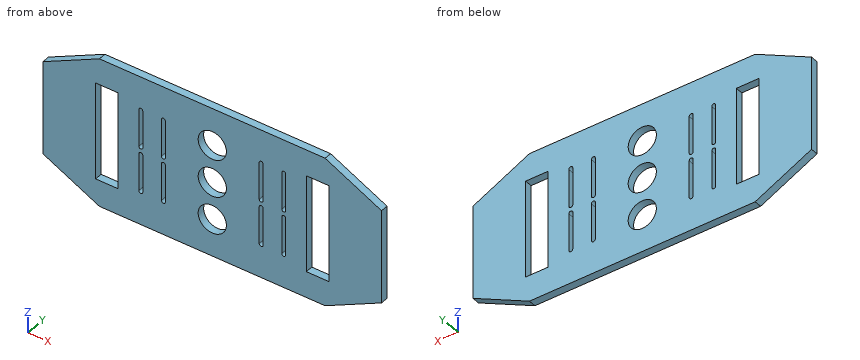
from build123d import *

# Parameters (mm, degrees)
ESQUISSE1_W             = 180
ESQUISSE1_H             = 80
BOSS_EXTRU_1_DEPTH      = 4
ENL_V_MAT_EXTRU_2_DEPTH = 4
ENL_V_MAT_EXTRU_3_DEPTH = 4
ENL_V_MAT_EXTRU_4_REACH = 6
ESQUISSE8_W             = 12
ESQUISSE8_H             = 52
ENL_V_MAT_EXTRU_5_REACH = 6
ESQUISSE9_R             = 7.5


with BuildPart() as part:
    # Esquisse1 → Boss.-Extru.1 (new body)
    with BuildSketch(Plane(origin=(0, 0, 0), x_dir=(1, 0, 0), z_dir=(0, 1, 0))):
        with Locations((90, 40)):
            Rectangle(ESQUISSE1_W, ESQUISSE1_H)
    extrude(amount=BOSS_EXTRU_1_DEPTH)

    # Esquisse2 → Enlèv. mat.-Extru.2 (cut)
    with BuildSketch(Plane(origin=(0, 4, 0), x_dir=(1, 0, 0), z_dir=(0, 1, 0))):
        Polygon((0, 65), (30, 80), (0, 80), align=None)
        Polygon((150, 80), (180, 65), (180, 80), align=None)
        Polygon((150, 0), (180, 15), (180, 0), align=None)
        Polygon((0, 15), (30, 0), (0, 0), align=None)
    extrude(amount=-ENL_V_MAT_EXTRU_2_DEPTH, mode=Mode.SUBTRACT)

    # Esquisse7 → Enlèv. mat.-Extru.3 (cut)
    with BuildSketch(Plane(origin=(0, 4, 0), x_dir=(1, 0, 0), z_dir=(0, 1, 0))):
        with BuildLine():
            Line((62.95, 18), (62.95, 38))
            ThreePointArc((62.95, 38), (64, 39.05), (65.05, 38))
            Line((65.05, 38), (65.05, 18))
            ThreePointArc((65.05, 18), (64, 16.95), (62.95, 18))
        make_face()
        with BuildLine():
            Line((50.95, 18), (50.95, 38))
            ThreePointArc((50.95, 38), (52, 39.05), (53.05, 38))
            Line((53.05, 38), (53.05, 18))
            ThreePointArc((53.05, 18), (52, 16.95), (50.95, 18))
        make_face()
        with BuildLine():
            Line((50.95, 42), (50.95, 62))
            ThreePointArc((50.95, 62), (52, 63.05), (53.05, 62))
            Line((53.05, 62), (53.05, 42))
            ThreePointArc((53.05, 42), (52, 40.95), (50.95, 42))
        make_face()
        with BuildLine():
            Line((62.95, 42), (62.95, 62))
            ThreePointArc((62.95, 62), (64, 63.05), (65.05, 62))
            Line((65.05, 62), (65.05, 42))
            ThreePointArc((65.05, 42), (64, 40.95), (62.95, 42))
        make_face()
        with BuildLine():
            Line((117.05, 42), (117.05, 62))
            ThreePointArc((117.05, 62), (116, 63.05), (114.95, 62))
            Line((114.95, 62), (114.95, 42))
            ThreePointArc((114.95, 42), (116, 40.95), (117.05, 42))
        make_face()
        with BuildLine():
            Line((129.05, 42), (129.05, 62))
            ThreePointArc((129.05, 62), (128, 63.05), (126.95, 62))
            Line((126.95, 62), (126.95, 42))
            ThreePointArc((126.95, 42), (128, 40.95), (129.05, 42))
        make_face()
        with BuildLine():
            Line((129.05, 18), (129.05, 38))
            ThreePointArc((129.05, 38), (128, 39.05), (126.95, 38))
            Line((126.95, 38), (126.95, 18))
            ThreePointArc((126.95, 18), (128, 16.95), (129.05, 18))
        make_face()
        with BuildLine():
            Line((117.05, 18), (117.05, 38))
            ThreePointArc((117.05, 38), (116, 39.05), (114.95, 38))
            Line((114.95, 38), (114.95, 18))
            ThreePointArc((114.95, 18), (116, 16.95), (117.05, 18))
        make_face()
    extrude(amount=-ENL_V_MAT_EXTRU_3_DEPTH, mode=Mode.SUBTRACT)

    # Esquisse8 → Enlèv. mat.-Extru.4 (cut, up to next)
    with BuildSketch(Plane(origin=(0, 4, 0), x_dir=(1, 0, 0), z_dir=(0, 1, 0)), mode=Mode.PRIVATE) as enl_v_mat_extru_4_sk1:
        with Locations((146, 40)):
            Rectangle(ESQUISSE8_W, ESQUISSE8_H)
    enl_v_mat_extru_4_tool1 = extrude(enl_v_mat_extru_4_sk1.sketch, amount=-ENL_V_MAT_EXTRU_4_REACH, mode=Mode.PRIVATE) & part.part
    add(enl_v_mat_extru_4_tool1.solids().sort_by_distance((146, 4, -40))[0], mode=Mode.SUBTRACT)
    # Esquisse8 → Enlèv. mat.-Extru.4 (cut, up to next)
    with BuildSketch(Plane(origin=(0, 4, 0), x_dir=(1, 0, 0), z_dir=(0, 1, 0)), mode=Mode.PRIVATE) as enl_v_mat_extru_4_sk2:
        with Locations((34, 40)):
            Rectangle(ESQUISSE8_W, ESQUISSE8_H)
    enl_v_mat_extru_4_tool2 = extrude(enl_v_mat_extru_4_sk2.sketch, amount=-ENL_V_MAT_EXTRU_4_REACH, mode=Mode.PRIVATE) & part.part
    add(enl_v_mat_extru_4_tool2.solids().sort_by_distance((34, 4, -40))[0], mode=Mode.SUBTRACT)

    # Esquisse9 → Enlèv. mat.-Extru.5 (cut, up to next)
    with BuildSketch(Plane.XZ, mode=Mode.PRIVATE) as enl_v_mat_extru_5_sk1:
        with Locations((90, -60)):
            Circle(ESQUISSE9_R)
    enl_v_mat_extru_5_tool1 = extrude(enl_v_mat_extru_5_sk1.sketch, amount=-ENL_V_MAT_EXTRU_5_REACH, mode=Mode.PRIVATE) & part.part
    add(enl_v_mat_extru_5_tool1.solids().sort_by_distance((90, 0, -60))[0], mode=Mode.SUBTRACT)
    # Esquisse9 → Enlèv. mat.-Extru.5 (cut, up to next)
    with BuildSketch(Plane.XZ, mode=Mode.PRIVATE) as enl_v_mat_extru_5_sk2:
        with Locations((90, -40)):
            Circle(ESQUISSE9_R)
    enl_v_mat_extru_5_tool2 = extrude(enl_v_mat_extru_5_sk2.sketch, amount=-ENL_V_MAT_EXTRU_5_REACH, mode=Mode.PRIVATE) & part.part
    add(enl_v_mat_extru_5_tool2.solids().sort_by_distance((90, 0, -40))[0], mode=Mode.SUBTRACT)
    # Esquisse9 → Enlèv. mat.-Extru.5 (cut, up to next)
    with BuildSketch(Plane.XZ, mode=Mode.PRIVATE) as enl_v_mat_extru_5_sk3:
        with Locations((90, -20)):
            Circle(ESQUISSE9_R)
    enl_v_mat_extru_5_tool3 = extrude(enl_v_mat_extru_5_sk3.sketch, amount=-ENL_V_MAT_EXTRU_5_REACH, mode=Mode.PRIVATE) & part.part
    add(enl_v_mat_extru_5_tool3.solids().sort_by_distance((90, 0, -20))[0], mode=Mode.SUBTRACT)


solid = part.part
Source: CAD feature listing. Evaluate the final solid. Frame: model axes, mm. Give positions to 0.01 mm unless a question says otherwise; leave off trailing zeros. Write each loop counter-clockwise with the first axis right and the second up, starting at its lowest first coordinate (ties: lowest second). Pieces come first, ordered by that corner, then holes. Notation, with made-up numbers: M -8.75,-3.5 L 35.25,-3.5 A8 cw 35.25,9.5 Z; hole C 18,78.25 d5. An arc over 180 degrees is marked long. Answer as a JSON object with one key per item and string values.
Q1. Cut plane A-A, the plane z = -25.5. Count the separate pieces of the cut face and the enclosed holes in it, then the cut area to 3 significant figures.
Geometry check:
{"separate pieces": "8", "enclosed holes": "0", "area": "550 mm^2"}
Q2. Cut plane B-B, the plane x = 167. Return the cut outline in (y, z).
Geometry check:
{"outline": "M 0,-71.5 L 4,-71.5 L 4,-8.5 L 0,-8.5 Z"}
Q3. Ray query, line 1 along Z through (x, y) = (90, 2.5); line 2 along Z through (x, y) = (92.5, 0.4); line 3 along Z through (x, y) = (64.5, 0.2). Return the intervals inside material, ascending.
Geometry check:
{"line 1": "z = -80 to -67.5, -52.5 to -47.5, -32.5 to -27.5, -12.5 to 0", "line 2": "z = -80 to -67.07, -52.93 to -47.07, -32.93 to -27.07, -12.93 to 0", "line 3": "z = -80 to -62.92, -41.08 to -38.92, -17.08 to 0"}
Q4. Contact query for flat-ended pins moving along their axis: P1, Ø1, axis at x = 155.5, y = 0.5, coming from the +Z side; P2, Ø1, axis at y = 2.5, z = -68.5, coming from the +X side. Output: stop coordinate, or through.
Geometry check:
{"P1": "stops at z = -2.5", "P2": "stops at x = 174"}
